Read the model definition and answer for the solid it produces. Units are mm, in the model's axes. A direction names the side the tool comes from. Round coordinates to 2 decimals unless told otherwise and drop trailing zeros. Order: outer loops, then holes, each group sorted by start corner. A loop starts at its lowest first (then second) coordinate and runs counter-clockwise, first axis right, second up. Notation, with made-up numbers: (83, 50) - (99, 50) arc R20 cw to (99, 67) - close; hole circle Ø6 at (5.5, 12.5). An arc over 180 degrees is marked (long way). Answer as a JSON object with one key per item and string values. Group by question number.
Q1. Consider line 1 (Y direction, x = -31.75, z = -6); line 2 (Y direction, x = -31.75, z = 10.5); line 3 (Z direction, x = -31, y = 1.75). Determine where each line is inside the solid, lowest interval first.
Q2. A cutting plane is placed at B-B on x = -31.75. Determine the outline of the cut face in (y, z), and give its area (3 significant figures).
Q3. Given pin 1 Ø1 at (x, y) = (-32, 1) entering from +Z; pin 2 Ø3.5 at (x, y) = (-31.5, 0) entering from -Z, each flat-ended and moving along its own axis, determine where each tip first touches the part or whether it passes through.
Q4. A cutting plane is placed at D-D on z = 1. Determine the outline of the cut face in (x, y).
Q5. A tool of negligible diameter and unlimited length cuts with its end or side. For faces 1 (the flat face through (-30, -1, 12.5)), 2 (the cylindrical face through (-29.656, -0.659, -4.049)), 3 (the cylindrical face through (-33.5, 0.08, 7.57)), from which of +Z, -Z, +X, -X, +Y, -Y can it reach the whole face along a straight path? Write none if from no direction.
Q6. A cutting plane is placed at C-C on y = -2. Determine the outline of the cut face in (x, z).
Q7. A cutting plane is placed at A-A on z = -2.5. Determine the outline of the cut face in (x, y).
Q8. The mould has two halves that part along Y. Classify faces 4 (the flat face through (-30, -2, -7.5)), 5 (the cylindrical face through (-34.924, -2.434, 2.36)), 6 (the flat face through (-32, 0, -0.5)): pulls with the +Y half, pulls with the -Y half, needs draft (parallel to the pull), parting line crosses it, or undercut.
```python
from build123d import *

# Parameters (mm, degrees)
SKETCH022_R     = 4
PAD009_DEPTH    = 20
SKETCH023_R     = 2.19496
POCKET011_DEPTH = 7
SKETCH025_R     = 1.75
POCKET012_DEPTH = 10


with BuildPart() as part:
    # Sketch022 → Pad009 (new body)
    with BuildSketch(Plane.XY):
        Circle(SKETCH022_R)
    extrude(amount=PAD009_DEPTH)

    # Sketch023 (on Face2 of Pad009) → Pocket011 (cut)
    with BuildSketch(Plane(origin=(0, 0, 0), x_dir=(1, 0, 0), z_dir=(0, 0, -1))):
        Circle(SKETCH023_R)
    extrude(amount=-POCKET011_DEPTH, mode=Mode.SUBTRACT)

    # Sketch025 (on Face3 of Pocket011) → Pocket012 (cut)
    with BuildSketch(Plane.XY.offset(20)):
        Circle(SKETCH025_R)
    extrude(amount=-POCKET012_DEPTH, mode=Mode.SUBTRACT)


with BuildPart() as part_1:
    # Body006 placement: moved
    add(part.part.moved(Location((-31.75, 0, -7.5))))


solid = part_1.part
```
Result set:
{
 "1": {"line 1": "y = -4 to -2.19, 2.19 to 4", "line 2": "y = -4 to -1.75, 1.75 to 4", "line 3": "z = -0.5 to 12.5"},
 "2": {"outline": "(-4, -7.5) - (-2.19, -7.5) - (-2.19, -0.5) - (2.19, -0.5) - (2.19, -7.5) - (4, -7.5) - (4, 12.5) - (1.75, 12.5) - (1.75, 2.5) - (-1.75, 2.5) - (-1.75, 12.5) - (-4, 12.5) - close", "area": "94.3 mm²"},
 "3": {"pin 1": "stops at z = 2.5", "pin 2": "stops at z = -0.5"},
 "4": {"outline": "circle Ø8 at (-31.75, 0)"},
 "5": {"face 1": "+Z, +X, -X, +Y, -Y", "face 2": "-Z", "face 3": "+Z"},
 "6": {"outline": "(-35.21, -7.5) - (-32.65, -7.5) - (-32.65, -0.5) - (-30.85, -0.5) - (-30.85, -7.5) - (-28.29, -7.5) - (-28.29, 12.5) - (-35.21, 12.5) - close"},
 "7": {"outline": "circle Ø8 at (-31.75, 0); hole circle Ø4.39 at (-31.75, 0)"},
 "8": {"face 4": "needs draft", "face 5": "parting line crosses it", "face 6": "undercut"}
}
